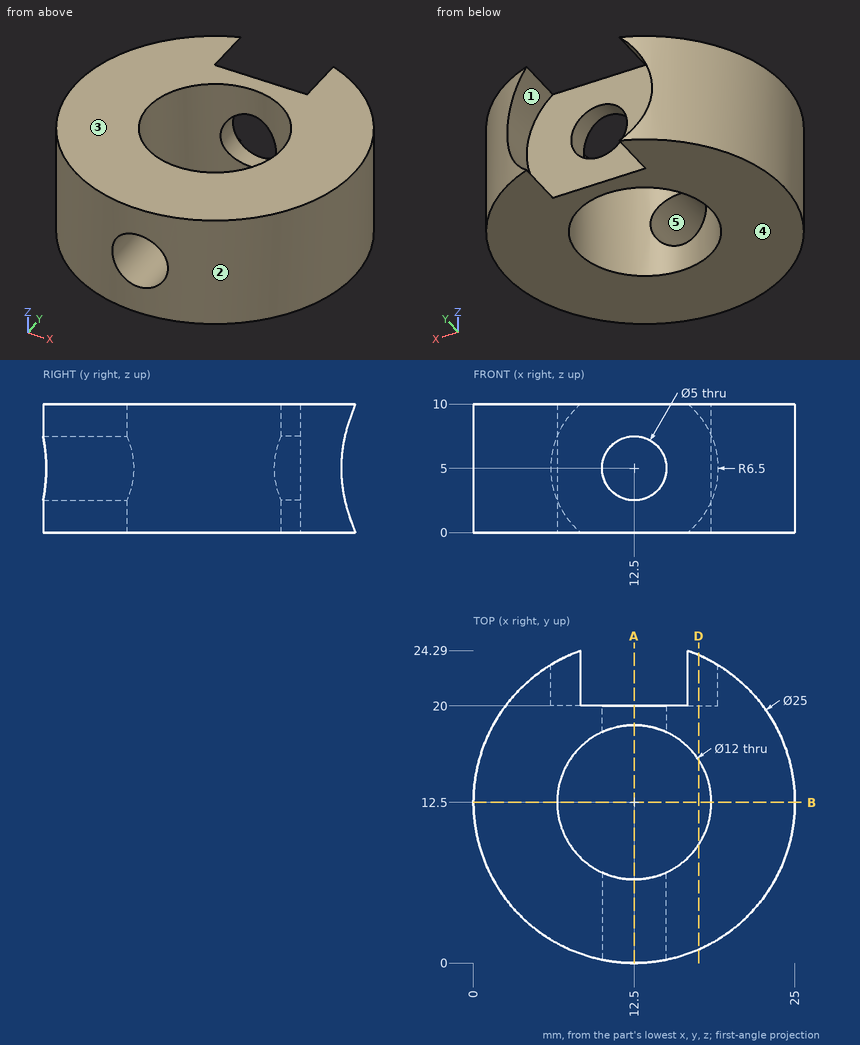
Print and shaded views of the part. All mm, measured from the part's lowest x, y and z. A direction names the side the tool comes from. Coordinates: 2 decimals unless noted, no trailing zeros. Loops run counter-clockwise (first coordinate to the right, second up) from the corner with the lowest first, then second, coordinate; pieces in that order, holes last. Notation, with made-up numbers: (-34.5, 67) -> (19.5, 67) arc R28 cw to (19.5, 95) -> close; hole circle Ø7 at (63.5, -32.5). An arc over 180 degrees is marked (long way). Use one line per item in the form item = value. Start each with the question number.
(1) Flat gauge pins, fed straight in: pin 1 (3 mm diameter, centred on y = 5, z = 2.5, fed in from -X); pin 2 (5 mm diameter, centred on y = 20.5, z = 4, fed in from -X) (3 decimals); pin 3 (3 mm diameter, centred on x = 12.5, z = 5, fed in from +Y); pin 4 (6 mm diameter, centred on y = 19.5, z = 5, fed in from -X). Where does each tip first touch, or does it go through?
(2) Cut at B-B on y = 12.5. Give the cut face in (x, z), and give its area (3 significant figures).
(3) Cut at D-D on x = 17.5. Give the cut face in (y, z).
(4) Tool access for the marked faces 1 and 2: list every direction of +Z, -Z, +X, -X, +Y, -Y with a clear straight run to the whole face (end or side of a thin tool).
(5) Cut at A-A on x = 12.5. Give the cut face in (y, z).
(6) Probe probe 1 along Z at (x, y) = (12.5, 4.75); probe 2 along X at (y, z) = (17.5, 5); probe 3 along X at (y, z) = (22.5, 2.25). List the from-to ranges inside material, lowest first. Write a range as from..to.
(7) Pull direction Z, two halves, no side cores. Call the marked faces 3, 4 and 5: pulls with the +Z half, pulls with the -Z half, needs draft (parallel to the pull), parting line crosses it, or undercut.
Values:
q1.pin_1 = 1.53
q1.pin_2 = 1.275
q1.pin_3 = through
q1.pin_4 = 0.66
q2.outline = (0, 0) -> (6.5, 0) -> (6.5, 10) -> (0, 10) -> close; (18.5, 0) -> (25, 0) -> (25, 10) -> (18.5, 10) -> close
q2.area = 130 mm2
q3.outline = (1.04, 0) -> (9.18, 0) -> (9.18, 10) -> (1.04, 10) -> close; (15.82, 0) -> (23.96, 0) -> (23.96, 0.85) -> (20, 0.85) -> (20, 9.15) -> (23.96, 9.15) -> (23.96, 10) -> (15.82, 10) -> close
q4.face_1 = +Y
q4.face_2 = +Z, -Z
q5.outline = (0, 0) -> (6.5, 0) -> (6.5, 2.5) -> (0, 2.5) -> close; (0, 7.5) -> (6.5, 7.5) -> (6.5, 10) -> (0, 10) -> close; (18.5, 0) -> (20, 0) -> (20, 2.5) -> (18.5, 2.5) -> close; (18.5, 7.5) -> (20, 7.5) -> (20, 10) -> (18.5, 10) -> close
q6.probe_1 = 0..2.5, 7.5..10
q6.probe_2 = 1.04..9.18, 15.82..23.96
q6.probe_3 = 5..6.61, 18.39..20
q7.face_3 = pulls with the +Z half
q7.face_4 = pulls with the -Z half
q7.face_5 = undercut
